```python
from build123d import *

# Parameters (mm, degrees)
EXTRUDE_1_DEPTH      = 2
EXTRUDE_1_DEPTH_BACK = 1
SKETCH_2_W           = 33.7
SKETCH_2_H           = 26.7
SKETCH_2_R           = 1.500160794
SKETCH_2_R_2         = 1.5
SKETCH_2_R_3         = 1.552324123
SKETCH_2_R_4         = 1.546482565
CUT_EXTRUDE_1_DEPTH  = 3
SKETCH_5_R           = 2.197988189
SKETCH_5_R_2         = 2.198876818
SKETCH_5_R_3         = 2.200287149
SKETCH_5_R_4         = 2.202466949
EXTRUDE_2_DEPTH      = 2.6
CUT_EXTRUDE_START    = -5
SKETCH_6_R           = 1.551176975
SKETCH_6_R_2         = 1.55471391
SKETCH_6_R_3         = 1.548240493
SKETCH_6_R_4         = 1.5
CUT_EXTRUDE_2_DEPTH  = 5
SKETCH_10_W          = 17.866024145
SKETCH_10_H          = 3.498646338
SKETCH_10_H_2        = 3.601530827
SKETCH_10_W_2        = 2.701736104
SKETCH_10_H_3        = 11.479623975
SKETCH_10_W_3        = 5.150482455
EXTRUDE_4_DEPTH      = 14
SKETCH_11_W          = 4.001103287
SKETCH_11_H          = 3.000250535
SKETCH_11_W_2        = 3.995812133
SKETCH_11_H_2        = 3
EXTRUDE_5_DEPTH      = 4.2
SKETCH_12_W          = 6.996994273
SKETCH_12_H          = 3.000250535
SKETCH_12_W_2        = 6.995985491
SKETCH_12_H_2        = 3
EXTRUDE_6_DEPTH      = 3
FILLET_4_R           = 3
FILLET_5_R           = 3
FILLET_6_R           = 3
FILLET_7_R           = 3


with BuildPart() as part:
    # Эскиз2 → Бобышка-Вытянуть1 (new, two sides: drawn at the far end of the back side and taken through both)
    with BuildSketch(Plane.XY.offset(-EXTRUDE_1_DEPTH_BACK)):
        with Locations((16.85, 13.35)):
            Rectangle(SKETCH_2_W, SKETCH_2_H)
        with Locations((30.998263896, 3.498646338)):
            Circle(SKETCH_2_R, mode=Mode.SUBTRACT)
        with Locations((30.998263896, 23.098469173)):
            Circle(SKETCH_2_R_2, mode=Mode.SUBTRACT)
        with Locations((5.150482455, 3.352746683)):
            Circle(SKETCH_2_R_3, mode=Mode.SUBTRACT)
        with Locations((5.150482455, 22.950000581)):
            Circle(SKETCH_2_R_4, mode=Mode.SUBTRACT)
    extrude(amount=EXTRUDE_1_DEPTH + EXTRUDE_1_DEPTH_BACK)

    # Эскиз4 → Вырез-Вытянуть1 (cut)
    with BuildSketch(Plane.XY.offset(2)):
        with BuildLine():
            Line((10.293463676, 5.094435071), (25.855282675, 5.094435071))
            ThreePointArc((25.855282675, 5.094435071), (27.976603018, 5.973114728), (28.855282675, 8.094435071))
            Line((28.855282675, 8.094435071), (28.855282675, 18.354211847))
            ThreePointArc((28.855282675, 18.354211847), (27.976603018, 20.475532191), (25.855282675, 21.354211847))
            Line((25.855282675, 21.354211847), (10.293463676, 21.354211847))
            ThreePointArc((10.293463676, 21.354211847), (8.172143332, 20.475532191), (7.293463676, 18.354211847))
            Line((7.293463676, 18.354211847), (7.293463676, 8.094435071))
            ThreePointArc((7.293463676, 8.094435071), (8.172143332, 5.973114728), (10.293463676, 5.094435071))
        make_face()
    extrude(amount=-CUT_EXTRUDE_1_DEPTH, mode=Mode.SUBTRACT)

    # Эскиз5 → Бобышка-Вытянуть2 (add)
    with BuildSketch(Plane.XY.offset(2)):
        with Locations(Location((5.150482455, 22.950000581, 0), (0, 0, 180))):
            Circle(SKETCH_5_R)
        with Locations(Location((30.998263896, 23.098469173, 0), (0, 0, 180))):
            Circle(SKETCH_5_R_2)
        with Locations(Location((30.998263896, 3.498646338, 0), (0, 0, 180))):
            Circle(SKETCH_5_R_3)
        with Locations(Location((5.150482455, 3.352746683, 0), (0, 0, 180))):
            Circle(SKETCH_5_R_4)
    extrude(amount=EXTRUDE_2_DEPTH)

    # Эскиз6 → Вырез-Вытянуть2 (cut)
    with BuildSketch(Plane.XY.offset(4.6).offset(CUT_EXTRUDE_START)):
        with Locations((5.150482455, 22.950000581)):
            Circle(SKETCH_6_R)
        with Locations((5.150482455, 3.352746683)):
            Circle(SKETCH_6_R_2)
        with Locations((30.998263896, 3.498646338)):
            Circle(SKETCH_6_R_3)
        with Locations((30.998263896, 23.098469173)):
            Circle(SKETCH_6_R_4)
    extrude(amount=CUT_EXTRUDE_2_DEPTH, mode=Mode.SUBTRACT)

    # Эскиз10 → Бобышка-Вытянуть4 (add)
    with BuildSketch(Plane(origin=(0, 0, -1), x_dir=(-1, 0, 0), z_dir=(0, 0, -1))):
        with Locations((-18.071569917, 1.749323169)):
            Rectangle(SKETCH_10_W, SKETCH_10_H)
        with Locations((-18.071569917, 24.899234587)):
            Rectangle(SKETCH_10_W, SKETCH_10_H_2)
        with Locations((-32.349131948, 13.292689749)):
            Rectangle(SKETCH_10_W_2, SKETCH_10_H_3)
        with Locations((-2.575241228, 13.292689749)):
            Rectangle(SKETCH_10_W_3, SKETCH_10_H_3)
    extrude(amount=EXTRUDE_4_DEPTH)

    # Эскиз11 → Бобышка-Вытянуть5 (add)
    with BuildSketch(Plane.XZ):
        with Locations((6.037312514, 0.499874732)):
            Rectangle(SKETCH_11_W, SKETCH_11_H)
        with Locations((27.668636997, 0.5)):
            Rectangle(SKETCH_11_W_2, SKETCH_11_H_2)
    extrude(amount=EXTRUDE_5_DEPTH)

    # Эскиз12 → Бобышка-Вытянуть6 (add)
    with BuildSketch(Plane.XZ.offset(4.2)):
        with Locations((6.037312514, 0.499874732)):
            Rectangle(SKETCH_12_W, SKETCH_12_H)
        with Locations((27.668636997, 0.5)):
            Rectangle(SKETCH_12_W_2, SKETCH_12_H_2)
    extrude(amount=EXTRUDE_6_DEPTH)

    # Скругление4
    fillet_4_edges = [part.edges().sort_by_distance(p)[0] for p in [
        (2.538815377, -7.2, 0.499874732),
    ]]
    fillet(fillet_4_edges, radius=FILLET_4_R - 0.0001)  # a hair under: the kernel refuses the full size

    # Скругление5
    fillet_5_edges = [part.edges().sort_by_distance(p)[0] for p in [
        (9.53580965, -7.2, 0.499874732),
    ]]
    fillet(fillet_5_edges, radius=FILLET_5_R - 0.0001)  # a hair under: the kernel refuses the full size

    # Скругление6
    fillet_6_edges = [part.edges().sort_by_distance(p)[0] for p in [
        (31.166629742, -7.2, 0.5),
    ]]
    fillet(fillet_6_edges, radius=FILLET_6_R - 0.0001)  # a hair under: the kernel refuses the full size

    # Скругление7
    fillet_7_edges = [part.edges().sort_by_distance(p)[0] for p in [
        (24.170644251, -7.2, 0.5),
    ]]
    fillet(fillet_7_edges, radius=FILLET_7_R - 0.0001)  # a hair under: the kernel refuses the full size


solid = part.part
```
Design review of the part built by this model. Coordinates are the model's own, in mm. A direction names the side the tool comes from. Coordinates: 2 decimals unless noted, no trailing zeros. Write each loop counter-clockwise with the first axis right and the second up, starting at its lowest first coordinate (ties: lowest second). Pieces come first, ordered by that corner, then holes.
1) Add section D-D (z = 0.5). State how many separate pieces and enclosed holes the cut face has, plus the area to 3 significant figures.
2) Mouldability with a two-part tool opening along Y and no side actions: class faces 4 (the flat face through (18, 2, -15)), 5 (the flat face through (3, 19.033, -8)), 6 (the cylindrical face through (28, 20.45, 0.52)) as +Y half, -Y half, draft (parallel to the pull), parting line (faces both ways), or undercut.
3) To check wall thickness, follow L1, parallel to Y at x = 21, z = -9.75; L2, parallel to X at y = 15, z = -11.5; L3, parallel to Y at x = 2, z = -0.5. State the ranges of each line that lie inside material, in increasing order.
4) Add section A-A (x = 23.5). Write out the cut boundary in (y, z).
5) Machinability: for faces 1 (the flat face through (18, 21.354, 1)), 2 (the flat face through (32, 19.033, -8)), 3 (the flat face through (27.005, 25, -8)), which of the approach directions +Z, -Z, +X, -X, +Y, -Y give a long, thin tool a straight path to every point of the face, cutting with its end or side? Answer none if there is none.
6) Insertion check: pin 1 (4 mm diameter, centred on x = 5.15, y = 22.95, fed in from -Z); pin 2 (2 mm diameter, centred on x = 7.5, z = -4.5, fed in from -Y); pin 3 (3.5 mm diameter, centred on x = 21, z = 1, fed in from -Y); pin 4 (2.5 mm diameter, centred on x = 2.5, z = -9, fed in from +Y). Each pin has a flat end and moves straight along its axis. Give the tip position at first contact, or say it passes through.
7) Add section B-B (y = 17). Write out the cut boundary in (x, z).
8) Add section C-C (z = -4.75). Write out the cut boundary in (x, y), plus the area to 3 significant figures.
Check result:
1. separate pieces: 1
1. enclosed holes: 5
1. area: 595 mm2
2. face 4: draft
2. face 5: +Y half
2. face 6: undercut
3. L1: y = 0 to 3.5, 23.1 to 26.7
3. L2: x = 0 to 5.15, 31 to 33.7
3. L3: y = 0 to 26.7
4. outline: (0, -15) - (3.5, -15) - (3.5, -1) - (5.09, -1) - (5.09, 2) - (0, 2) - close; (21.35, -1) - (23.1, -1) - (23.1, -15) - (26.7, -15) - (26.7, 2) - (21.35, 2) - close
5. face 1: +Z, -Z
5. face 2: -Z, +X, -X, +Y
5. face 3: -Z, +X, +Y, -Y
6. pin 1: stops at z = -1
6. pin 2: passes through
6. pin 3: stops at y = 0
6. pin 4: stops at y = 19.03
7. outline: (0, -15) - (5.15, -15) - (5.15, -1) - (7.29, -1) - (7.29, 2) - (0, 2) - close; (28.86, -1) - (31, -1) - (31, -15) - (33.7, -15) - (33.7, 2) - (28.86, 2) - close
8. outline: (0, 7.55) - (5.15, 7.55) - (5.15, 19.03) - (0, 19.03) - close; (9.14, 0) - (27, 0) - (27, 3.5) - (9.14, 3.5) - close; (9.14, 23.1) - (27, 23.1) - (27, 26.7) - (9.14, 26.7) - close; (31, 7.55) - (33.7, 7.55) - (33.7, 19.03) - (31, 19.03) - close
8. area: 217 mm2
